```python
from build123d import *

# Parameters (mm, degrees)
ESQUISSE1_W                = 250
ESQUISSE1_H                = 130
BOSS_EXTRU_1_DEPTH         = 3.175
ESQUISSE2_W                = 10
ESQUISSE2_H                = 3.175
BOSS_EXTRU_2_DEPTH         = 3.175
R_P_TITION_LIN_AIRE1_COUNT = 12
R_P_TITION_LIN_AIRE1_PITCH = 20
ESQUISSE3_W                = 3.175
ESQUISSE3_H                = 10
BOSS_EXTRU_3_DEPTH         = 3.175
R_P_TITION_LIN_AIRE2_COUNT = 6
R_P_TITION_LIN_AIRE2_PITCH = 20


with BuildPart() as part:
    # Esquisse1 → Boss.-Extru.1 (new body)
    with BuildSketch(Plane(origin=(0, 0, 0), x_dir=(1, 0, 0), z_dir=(0, 1, 0))):
        with Locations((125, 65)):
            Rectangle(ESQUISSE1_W, ESQUISSE1_H)
    extrude(amount=BOSS_EXTRU_1_DEPTH)

    # Esquisse2 → Boss.-Extru.2 (add)
    with BuildSketch(Plane(origin=(0, 3.175, 0), x_dir=(1, 0, 0), z_dir=(0, 1, 0))):
        with Locations((15, 131.5875)):
            Rectangle(ESQUISSE2_W, ESQUISSE2_H)
        with Locations((15, -1.5875)):
            Rectangle(ESQUISSE2_W, ESQUISSE2_H)
    boss_extru_2 = extrude(amount=-BOSS_EXTRU_2_DEPTH)

    # Répétition linéaire1: Boss.-Extru.2 ×12
    with Locations(*[(i * R_P_TITION_LIN_AIRE1_PITCH, 0, 0) for i in range(1, R_P_TITION_LIN_AIRE1_COUNT)]):
        add(boss_extru_2)

    # Esquisse3 → Boss.-Extru.3 (add)
    with BuildSketch(Plane(origin=(0, 3.175, 0), x_dir=(1, 0, 0), z_dir=(0, 1, 0))):
        with Locations((251.5875, 115)):
            Rectangle(ESQUISSE3_W, ESQUISSE3_H)
        with Locations((-1.5875, 115)):
            Rectangle(ESQUISSE3_W, ESQUISSE3_H)
    boss_extru_3 = extrude(amount=-BOSS_EXTRU_3_DEPTH)

    # Répétition linéaire2: Boss.-Extru.3 ×6
    with Locations(*[(0, 0, i * R_P_TITION_LIN_AIRE2_PITCH) for i in range(1, R_P_TITION_LIN_AIRE2_COUNT)]):
        add(boss_extru_3)


solid = part.part
```
CAD build for the part. Positions are in the model's coordinates, mm. Round coordinates to 2 decimals unless told otherwise and drop trailing zeros. Order: outer loops, then holes, each group sorted by start corner. A loop starts at its lowest first (then second) coordinate and runs counter-clockwise, first axis right, second up.
Item 1: Probe line 1 along X through (y, z) = (1.9, -42.5); line 2 along Z through (x, y) = (169, 0.95). List the from-to ranges inside material, lowest first.
Item 2: Pin check, flat tips, straight feed: pin 1 (1 mm diameter, centred on y = 1, z = -132, fed in from -X); pin 2 (1 mm diameter, centred on y = 2, z = -47, fed in from -X); pin 3 (1 mm diameter, centred on y = 1, z = -6.5, fed in from +X). Stop position of each tip, or through.
Item 3: Saw through at B-B on x = 144. Write the cut outline in (y, z) (3 decimals).
Item 4: Saw through at A-A on z = -83.5. Write the cut outline in (x, y) (3 decimals), then the cut area to 3 significant figures.
Reported:
1. line 1: x = 0 to 250
1. line 2: z = -130 to 0
2. pin 1: stops at x = 10
2. pin 2: stops at x = 0
2. pin 3: stops at x = 250
3. outline: (0, -130) - (3.175, -130) - (3.175, 0) - (0, 0) - close
4. outline: (0, 0) - (250, 0) - (250, 3.175) - (0, 3.175) - close
4. area: 794 mm2
